Work out the finished part from the listing and answer in its coordinate system (mm). Give positions to 0.01 mm unless a question says otherwise; leave off trailing zeros. Loops run counter-clockwise (first coordinate to the right, second up) from the corner with the lowest first, then second, coordinate; pieces in that order, holes last. Notation, with made-up numbers: M -32.5,86 L -21.5,86 A22 cw -21.5,94 Z; hole C 9,-3.75 d7. An arc over 180 degrees is marked long. Use a Markdown table: item, result.
```python
from build123d import *

# Parameters (mm, degrees)
BOSS_EXTRUDE1_DEPTH                                 = 5
CBORE_FOR_M8_HEX_SOCKET_HEAD_CAP_SCREW1_D           = 9
CBORE_FOR_M8_HEX_SOCKET_HEAD_CAP_SCREW1_CBORE_D     = 15
CBORE_FOR_M8_HEX_SOCKET_HEAD_CAP_SCREW1_CBORE_DEPTH = 8.6
SKETCH5_R                                           = 11
CUT_EXTRUDE2_DEPTH                                  = 465.569693372
CBORE_FOR_M3_HEX_SOCKET_HEAD_CAP_SCREW1_D           = 3.4
CBORE_FOR_M3_HEX_SOCKET_HEAD_CAP_SCREW1_CBORE_D     = 6.5
CBORE_FOR_M3_HEX_SOCKET_HEAD_CAP_SCREW1_CBORE_DEPTH = 3.4
FILLET1_R                                           = 25
M10_CLEARANCE_HOLE1_D                               = 11
M10_CLEARANCE_HOLE1_DEPTH                           = 25
M10_CLEARANCE_HOLE1_TIP                             = 3.304733405


with BuildPart() as part:
    # Sketch1 → Boss-Extrude1 (new, symmetric)
    with BuildSketch(Plane.XY):
        Polygon((-115, 200), (-115, 0), (115, 0), (115, 450), (15, 450), align=None)
    extrude(amount=BOSS_EXTRUDE1_DEPTH, both=True)

    # CBORE for M8 Hex Socket Head Cap Screw1 (through all)
    with Locations(Plane.XY.offset(5)):
        with Locations((-90, 17.5), (-45, 17.5), (45, 17.5), (90, 17.5), (0, 17.5), (-90, 62.5), (-45, 62.5), (45, 62.5), (90, 62.5), (0, 62.5)):
            CounterBoreHole(CBORE_FOR_M8_HEX_SOCKET_HEAD_CAP_SCREW1_D / 2, CBORE_FOR_M8_HEX_SOCKET_HEAD_CAP_SCREW1_CBORE_D / 2, CBORE_FOR_M8_HEX_SOCKET_HEAD_CAP_SCREW1_CBORE_DEPTH)

    # Sketch5 → Cut-Extrude2 (cut, through all)
    with BuildSketch(Plane.XY.offset(5)):
        with Locations((93.85, 428.85)):
            Circle(SKETCH5_R)
    extrude(amount=-CUT_EXTRUDE2_DEPTH, mode=Mode.SUBTRACT)

    # CBORE for M3 Hex Socket Head Cap Screw1 (through all)
    with Locations(Plane(origin=(0, 0, -5), x_dir=(1, 0, 0), z_dir=(0, 0, -1))):
        with Locations((109.35, -444.35), (78.35, -444.35), (78.35, -413.35), (109.35, -413.35)):
            CounterBoreHole(CBORE_FOR_M3_HEX_SOCKET_HEAD_CAP_SCREW1_D / 2, CBORE_FOR_M3_HEX_SOCKET_HEAD_CAP_SCREW1_CBORE_D / 2, CBORE_FOR_M3_HEX_SOCKET_HEAD_CAP_SCREW1_CBORE_DEPTH)

    # Fillet1
    fillet1_edges = [part.edges().sort_by_distance(p)[0] for p in [
        (-115, 200, 0),
        (15, 450, 0),
    ]]
    fillet(fillet1_edges, radius=FILLET1_R)

    # M10 Clearance Hole1
    with Locations(Plane.XY.offset(5)):
        with Locations((92.5, 387.5), (92.5, 342.5)):
            Hole(M10_CLEARANCE_HOLE1_D / 2, depth=M10_CLEARANCE_HOLE1_DEPTH)
            with Locations((0, 0, -(M10_CLEARANCE_HOLE1_DEPTH + M10_CLEARANCE_HOLE1_TIP / 2))):  # 118° drill point
                Cone(0, M10_CLEARANCE_HOLE1_D / 2, M10_CLEARANCE_HOLE1_TIP, mode=Mode.SUBTRACT)


solid = part.part
```
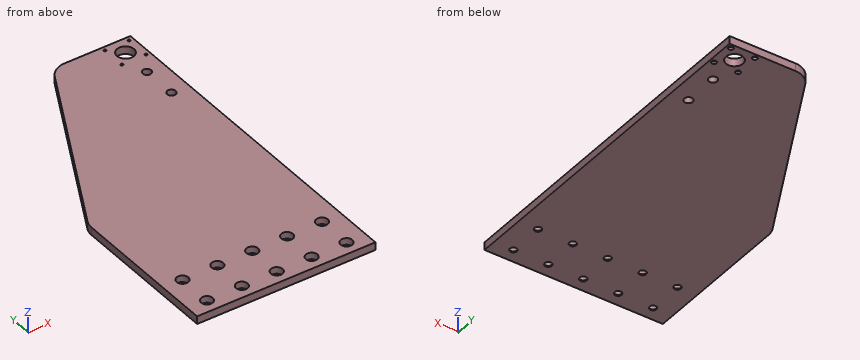
(1) A cutting plane is placed at D-D (y = 240). Write down the section's boundary in (x, z).
Entries:
| item | result |
|---|---|
| outline | M -94.2,-5 L 115,-5 L 115,5 L -94.2,5 Z |
(2) A cutting plane is placed at A-A (y = 387.5). Write down the section's boundary in (x, z), and give its area (4 significant figures).
Entries:
| item | result |
|---|---|
| outline | M -17.5,-5 L 87,-5 L 87,5 L -17.5,5 Z; M 98,-5 L 115,-5 L 115,5 L 98,5 Z |
| area | 1,215 mm² |
(3) Given P1, Ø2, axis at x = -72, z = -2, coming from the +Y side; P2, Ø4.5, axis at x = -46.5, y = 59.5, coming from the +Z side; P3, Ø4, axis at x = -14, z = -4, coming from the +Y side, each flat-ended and moving along its own axis, determine where each tip first touches the part or whether it passes through.
Entries:
| item | result |
|---|---|
| P1 | stops at y = 284.62 |
| P2 | stops at z = -3.6 |
| P3 | stops at y = 398.08 |
(4) Consider probe 1 along Y at (x, z) = (109.35, 3); probe 2 along Y at (x, z) = (44, 2.75); probe 3 along Y at (x, z) = (90, -0.5). Determine where each line is inside the solid, lowest interval first. Write a range as [from, to].
Entries:
| item | result |
|---|---|
| probe 1 | y = [0, 411.65], [415.05, 442.65], [446.05, 450] |
| probe 2 | y = [0, 10.07], [24.93, 55.07], [69.93, 450] |
| probe 3 | y = [0, 10], [25, 55], [70, 337.6], [347.4, 382.6], [392.4, 418.55], [439.15, 450] |
(5) A cutting plane is placed at C-C (x = -45). Write down the section's boundary in (y, z).
Entries:
| item | result |
|---|---|
| outline | M 0,-5 L 13,-5 L 13,-3.6 L 10,-3.6 L 10,5 L 0,5 Z; M 22,-5 L 58,-5 L 58,-3.6 L 55,-3.6 L 55,5 L 25,5 L 25,-3.6 L 22,-3.6 Z; M 67,-5 L 334.62,-5 L 334.62,5 L 70,5 L 70,-3.6 L 67,-3.6 Z |
(6) A cutting plane is placed at B-B (z = 1). Count the separate pieces of the cut face and the enclosed holes in it, and give its area (3 significant figures).
Entries:
| item | result |
|---|---|
| separate pieces | 1 |
| enclosed holes | 17 |
| area | 84,800 mm² |
